The listing builds one solid part. Answer for the finished solid, in the listing's coordinates (mm). A direction names the side the tool comes from. Coordinates: 2 decimals unless noted, no trailing zeros. Loops run counter-clockwise (first coordinate to the right, second up) from the corner with the lowest first, then second, coordinate; pieces in that order, holes last. Notation, with made-up numbers: M -15,68 L -5,68 A13 ccw -5,85 Z; hole C -23.75,-9 d4. An arc over 180 degrees is marked long. Answer as CSV lines item,"result". Start each with the question number.
```python
from build123d import *

# Parameters (mm, degrees)
BASE_W                              = 36
BASE_H                              = 30
BOSS_EXTRUDE1_DEPTH                 = 4.5
WALLS_W                             = 36
WALLS_H                             = 5
WALLS_EXT_DEPTH                     = 31.5
SWITCH_BLOCK_W                      = 15
SWITCH_BLOCK_H                      = 30
SWITCH_BLOCK_EXT_DEPTH              = 15.25
MAGNET_POCKET_R                     = 6.25
MAGNET_POCKET_CUT_DEPTH             = 3.75
FILLET1_R                           = 5
FILLET2_R                           = 5
FILLET3_R                           = 20
FILLET4_R                           = 20
SWITCH_PLACE_W                      = 14
SWITCH_PLACE_H                      = 6.1
SWITCH_POCKET_DEPTH                 = 5.25
SWITCH_CONTACTS_W                   = 14
SWITCH_CONTACTS_H                   = 2.5
SWITCH_LEADS_DEPTH                  = 7
SWITCH_ANGLE_LEFT_DEPTH             = 1.8
SWITCH_ANGLE_RIGHT_DEPTH            = 1.8
SKETCH20_W                          = 8.1
SKETCH20_H                          = 12
BOSS_EXTRUDE5_DEPTH                 = 1
FILLET5_R                           = 1
FILLET6_R                           = 1
WIRE_GUIDE_W                        = 8
WIRE_GUIDE_H                        = 4
WIRE_PASS_THROUGH_DEPTH             = 7.5
WIRE_PASS_THROUGH_DIRECTION_2_REACH = 38.056
WIRE_CHANNEL_OUTLINE_W              = 4
WIRE_CHANNEL_OUTLINE_H              = 4
WIRE_CHANNEL_DEPTH                  = 1.5
ACHSE_R                             = 1.1
M2_ACHSE_DEPTH                      = 55.002314765
M2_NUT_DEPTH                        = 2.5
SKETCH2_R                           = 1.575
M3_MOUNTING_SCREWS_DEPTH            = 4.5
SKETCH9_W                           = 2
SKETCH9_H                           = 2
BOSS_EXTRUDE3_DEPTH                 = 11.95
SKETCH10_W                          = 2
SKETCH10_H                          = 2
BOSS_EXTRUDE4_DEPTH                 = 11.95
SKETCH19_R                          = 2
SCREW_HEAD_DEPTH                    = 2
SKETCH21_W                          = 21
SKETCH21_H                          = 27
CUT_EXTRUDE2_DEPTH                  = 0.25
SKETCH22_W                          = 21
SKETCH22_H                          = 27
CUT_EXTRUDE3_DEPTH                  = 0.25


# Read off the part's stored shape, not the designer's step: Wire Channel
with BuildPart() as part:
    # Base → Boss-Extrude1 (new body)
    with BuildSketch(Plane(origin=(0, 0, 0), x_dir=(1, 0, 0), z_dir=(0, 1, 0))):
        Rectangle(BASE_W, BASE_H)
    extrude(amount=BOSS_EXTRUDE1_DEPTH)

    # Walls → Walls Ext (add)
    with BuildSketch(Plane.XZ):
        with Locations((0, 17.5)):
            Rectangle(WALLS_W, WALLS_H)
        with Locations((0, -17.5)):
            Rectangle(WALLS_W, WALLS_H)
    extrude(amount=-WALLS_EXT_DEPTH)

    # Switch Block → Switch Block Ext (add)
    with BuildSketch(Plane(origin=(0, 4.5, 0), x_dir=(1, 0, 0), z_dir=(0, 1, 0))):
        with Locations((-10.5, 0)):
            Rectangle(SWITCH_BLOCK_W, SWITCH_BLOCK_H)
    extrude(amount=SWITCH_BLOCK_EXT_DEPTH)

    # Magnet Pocket → Magnet Pocket Cut (cut)
    with BuildSketch(Plane(origin=(0, 0, 0), x_dir=(1, 0, 0), z_dir=(0, 1, 0))):
        with Locations(Location((10, 0, 0), (0, 0, 90))):
            Circle(MAGNET_POCKET_R)
    extrude(amount=MAGNET_POCKET_CUT_DEPTH, mode=Mode.SUBTRACT)

    # Fillet1
    fillet1_edges = [part.edges().sort_by_distance(p)[0] for p in [
        (-18, 31.5, -17.5),
    ]]
    fillet(fillet1_edges, radius=FILLET1_R)

    # Fillet2
    fillet2_edges = [part.edges().sort_by_distance(p)[0] for p in [
        (-18, 31.5, 17.5),
    ]]
    fillet(fillet2_edges, radius=FILLET2_R)

    # Fillet3
    fillet3_edges = [part.edges().sort_by_distance(p)[0] for p in [
        (18, 31.5, -17.5),
    ]]
    fillet(fillet3_edges, radius=FILLET3_R)

    # Fillet4
    fillet4_edges = [part.edges().sort_by_distance(p)[0] for p in [
        (18, 31.5, 17.5),
    ]]
    fillet(fillet4_edges, radius=FILLET4_R)

    # Switch Place → Switch Pocket (cut)
    with BuildSketch(Plane(origin=(0, 19.75, 0), x_dir=(1, 0, 0), z_dir=(0, 1, 0))):
        with Locations((-10, 0)):
            Rectangle(SWITCH_PLACE_W, SWITCH_PLACE_H)
    extrude(amount=-SWITCH_POCKET_DEPTH, mode=Mode.SUBTRACT)

    # Switch Contacts → Switch Leads (cut)
    with BuildSketch(Plane(origin=(0, 14.5, 0), x_dir=(1, 0, 0), z_dir=(0, 1, 0))):
        with Locations((-10, 0)):
            Rectangle(SWITCH_CONTACTS_W, SWITCH_CONTACTS_H)
    extrude(amount=-SWITCH_LEADS_DEPTH, mode=Mode.SUBTRACT)

    # Sketch16 → Switch Angle Left (add)
    with BuildSketch(Plane(origin=(0, 0, 3.05), x_dir=(-1, 0, 0), z_dir=(0, 0, -1))):
        Polygon((17, 14.5), (17, 14.75), (3, 14.5), align=None)
    extrude(amount=SWITCH_ANGLE_LEFT_DEPTH)

    # Sketch17 → Switch Angle Right (add)
    with BuildSketch(Plane.XY.offset(-3.05)):
        Polygon((-17, 14.5), (-17, 14.75), (-3, 14.5), align=None)
    extrude(amount=SWITCH_ANGLE_RIGHT_DEPTH)

    # Sketch20 → Boss-Extrude5 (add)
    with BuildSketch(Plane(origin=(-3, 0, 0), x_dir=(0, 0, -1), z_dir=(1, 0, 0))):
        with Locations((0, 10.5)):
            Rectangle(SKETCH20_W, SKETCH20_H)
    extrude(amount=BOSS_EXTRUDE5_DEPTH)

    # Fillet5
    fillet5_edges = [part.edges().sort_by_distance(p)[0] for p in [
        (-2, 10.5, 4.05),
    ]]
    fillet(fillet5_edges, radius=FILLET5_R - 0.0001)  # a hair under: the kernel refuses the full size

    # Fillet6
    fillet6_edges = [part.edges().sort_by_distance(p)[0] for p in [
        (-2, 10.5, -4.05),
    ]]
    fillet(fillet6_edges, radius=FILLET6_R - 0.0001)  # a hair under: the kernel refuses the full size

    # Wire Guide → Wire pass through (cut)
    with BuildSketch(Plane(origin=(0, 7.5, 0), x_dir=(1, 0, 0), z_dir=(0, 1, 0))):
        with Locations((-10, 0)):
            Rectangle(WIRE_GUIDE_W, WIRE_GUIDE_H)
    extrude(amount=-WIRE_PASS_THROUGH_DEPTH, mode=Mode.SUBTRACT)

    # Wire pass through direction 2: up to this plane
    wire_pass_through_direction_2_end = Plane(origin=(-17, 14.75, -12.752231965), z_dir=(-0.017854296416882947, -0.9998405993454447, 0))
    # Wire Guide → Wire pass through direction 2 (cut, up to the surface)
    with BuildSketch(Plane(origin=(0, 7.5, 0), x_dir=(1, 0, 0), z_dir=(0, 1, 0)), mode=Mode.PRIVATE) as wire_pass_through_direction_2_sk1:
        with Locations((-10, 0)):
            Rectangle(WIRE_GUIDE_W, WIRE_GUIDE_H)
    wire_pass_through_direction_2_tool1 = split(extrude(wire_pass_through_direction_2_sk1.sketch, amount=WIRE_PASS_THROUGH_DIRECTION_2_REACH, mode=Mode.PRIVATE), bisect_by=wire_pass_through_direction_2_end, keep=Keep.BOTH, mode=Mode.PRIVATE)
    add(wire_pass_through_direction_2_tool1.solids().sort_by_distance((-10, 7.5, 0))[0], mode=Mode.SUBTRACT)

    # Wire Channel outline → Wire Channel (cut)
    with BuildSketch(Plane(origin=(0, 0, 0), x_dir=(1, 0, 0), z_dir=(0, 1, 0))):
        with Locations((-16, 0)):
            Rectangle(WIRE_CHANNEL_OUTLINE_W, WIRE_CHANNEL_OUTLINE_H)
        with BuildLine():
            Line((-6, 2), (-6, -2))
            Line((-6, -2), (0.968804066, -2))
            ThreePointArc((0.968804066, -2), (0.75, 0), (0.968804066, 2))
            Line((0.968804066, 2), (-6, 2))
        make_face()
    extrude(amount=WIRE_CHANNEL_DEPTH, mode=Mode.SUBTRACT)

    # Achse → M2 Achse (cut, through all)
    with BuildSketch(Plane.XY.offset(20)):
        with Locations((-10, 25.5)):
            Circle(ACHSE_R)
    extrude(amount=-M2_ACHSE_DEPTH, mode=Mode.SUBTRACT)

    # Sketch5 → M2 Nut (cut)
    with BuildSketch(Plane(origin=(0, 0, -20), x_dir=(-1, 0, 0), z_dir=(0, 0, -1))):
        Polygon((10, 27.6), (8.181346652, 26.55), (8.181346652, 24.45), (10, 23.4), (11.818653348, 24.45), (11.818653348, 26.55), align=None)
    extrude(amount=-M2_NUT_DEPTH, mode=Mode.SUBTRACT)

    # Sketch2 → M3 Mounting Screws (cut)
    with BuildSketch(Plane.XZ):
        with Locations(Location((2, -10, 0), (0, 0, 270))):
            Circle(SKETCH2_R)
        with Locations(Location((2, 10, 0), (0, 0, 270))):
            Circle(SKETCH2_R)
    extrude(amount=-M3_MOUNTING_SCREWS_DEPTH, mode=Mode.SUBTRACT)

    # M3 Senkkopf cone 1 section (through the dimple's axis) → M3 Senkkopf (revolve, cut)
    with BuildSketch(Plane(origin=(2, 4.5, 10), x_dir=(0, 0, 1), z_dir=(1, 0, 0))):
        Polygon((0, 0), (3.25, 0), (0, 3.25), align=None)
    revolve(axis=Axis((2, 4.5, 10), (0, -1, 0)), mode=Mode.SUBTRACT)

    # M3 Senkkopf cone 2 section (through the dimple's axis) → M3 Senkkopf cone 2 (revolve, cut)
    with BuildSketch(Plane(origin=(2, 4.5, -10), x_dir=(0, 0, 1), z_dir=(1, 0, 0))):
        Polygon((0, 0), (3.25, 0), (0, 3.25), align=None)
    revolve(axis=Axis((2, 4.5, -10), (0, -1, 0)), mode=Mode.SUBTRACT)

    # Sketch9 → Boss-Extrude3 (add)
    with BuildSketch(Plane.XY.offset(-15)):
        with Locations((-17, 20.75)):
            Rectangle(SKETCH9_W, SKETCH9_H)
    extrude(amount=BOSS_EXTRUDE3_DEPTH)

    # Sketch10 → Boss-Extrude4 (add)
    with BuildSketch(Plane(origin=(0, 0, 15), x_dir=(-1, 0, 0), z_dir=(0, 0, -1))):
        with Locations((17, 20.75)):
            Rectangle(SKETCH10_W, SKETCH10_H)
    extrude(amount=BOSS_EXTRUDE4_DEPTH)

    # Sketch19 → Screw Head (cut)
    with BuildSketch(Plane.XY.offset(20)):
        with Locations((-10, 25.5)):
            Circle(SKETCH19_R)
    extrude(amount=-SCREW_HEAD_DEPTH, mode=Mode.SUBTRACT)

    # Sketch21 → Cut-Extrude2 (cut)
    with BuildSketch(Plane(origin=(0, 0, 15), x_dir=(-1, 0, 0), z_dir=(0, 0, -1))):
        with Locations((-7.5, 18)):
            Rectangle(SKETCH21_W, SKETCH21_H)
    extrude(amount=-CUT_EXTRUDE2_DEPTH, mode=Mode.SUBTRACT)

    # Sketch22 → Cut-Extrude3 (cut)
    with BuildSketch(Plane.XY.offset(-15)):
        with Locations((7.5, 18)):
            Rectangle(SKETCH22_W, SKETCH22_H)
    extrude(amount=-CUT_EXTRUDE3_DEPTH, mode=Mode.SUBTRACT)


solid = part.part
```
Item 1: Each of these flat-tipped pins is pushed along its axis until it touches: P1, Ø3, axis at y = 8, z = 1, coming from the +X side; P2, Ø11, axis at x = 10, z = 0, coming from the +Y side; P3, Ø1, axis at y = 20.5, z = 8.5, coming from the +X side. Where does it stop, or does it pass through?
Item 2: Consider line 1 (Z direction, x = 2, y = 1) (3 decimals); line 2 (X direction, y = 1.5, z = -10) (3 decimals); line 3 (Z direction, x = -14.5, y = 18). Determine where each line is inside the solid, lowest interval first.
Item 3: Section B-B on y = 25.5 is taken. Determine the outline of the cut face in (x, z), then the cut area to 3 significant figures.
Item 4: Section A-A on z = -10 is taken. Determine the outline of the cut face in (x, y) (3 decimals).
Item 5: Section C-C on x = -10.5 is taken. State how many separate pieces and enclosed holes the cut face has, then the cut area to 3 significant figures.
Item 6: For faces 4 (the face through (-4, 11, -1.25)), 5 (the face through (-14, 7, 0)), 6 (the face through (-2.301, 10.584, 3.765)), 7 (the face through (-9.1, 24.6, 18)), determine the directions among +Z, -Z, +X, -X, +Y, -Y from which every point of the face is accessible in a straight line to the end or side of a thin tool.
Item 7: For a pull along Y with two mould halves and no side action, classify faces 1 (the face through (-10, 24, -17.5)), 2 (the face through (-15, 11, -1.25)), 3 (the face through (-2.5, 16.5, 0.1)) as pulls with the +Y half, pulls with the -Y half, needs draft (parallel to the pull), parting line crosses it, or undercut.
Results are:
1,P1,"x = -2"
1,P2,"y = 4.5"
1,P3,"x = -16"
2,line 1,"-20 to -11.575, -8.425 to 8.425, 11.575 to 20"
2,line 2,"-18 to 0.425, 3.575 to 18"
2,line 3,"-20 to -3.05, 3.05 to 20"
3,outline,"M -18,-20 L -11.82,-20 L -11.82,-17.5 L -11.1,-17.5 L -11.1,-15 L -18,-15 Z; M -18,15 L -11.1,15 L -11.1,18 L -12,18 L -12,20 L -18,20 Z; M -8.9,-17.5 L -8.18,-17.5 L -8.18,-20 L 12.28,-20 L 12.28,-15.25 L -3,-15.25 L -3,-15 L -8.9,-15 Z; M -8.9,15 L -3,15 L -3,15.25 L 12.28,15.25 L 12.28,20 L -8,20 L -8,18 L -8.9,18 Z"
3,area,"266 mm²"
4,outline,"M -18,0 L 0.425,0 L 0.425,2.825 L -1.25,4.5 L -3,4.5 L -3,19.75 L -16,19.75 L -16,21.75 L -18,21.75 Z; M 3.575,0 L 18,0 L 18,4.5 L 5.25,4.5 L 3.575,2.825 Z"
5,separate pieces,"4"
5,enclosed holes,"0"
5,area,"790 mm²"
6,face 4,"+Y"
6,face 5,"+Y, -Y"
6,face 6,"+X, +Y"
6,face 7,"+Z"
7,face 1,"undercut"
7,face 2,"needs draft"
7,face 3,"pulls with the +Y half"
